Source: CAD feature listing. Evaluate the final solid. Frame: model axes, mm. A direction names the side the tool comes from. Round coordinates to 2 decimals unless told otherwise and drop trailing zeros. Order: outer loops, then holes, each group sorted by start corner. A loop starts at its lowest first (then second) coordinate and runs counter-clockwise, first axis right, second up. Notation, with made-up numbers: (79, 79.25) -> (101, 79.25) arc R26 ccw to (101, 109.25) -> close; hole circle Ø7 at (1.25, 48.5). An arc over 180 degrees is marked (long way). Use a Markdown table: item, result. Add a question column.
Autodesk Inventor part; units mm, degrees
ref_plane "YZ Plane" through (0, 0, 0) normal (1, 0, 0) x (0, 1, 0)
ref_plane "XZ Plane" through (0, 0, 0) normal (0, 1, 0) x (-1, 0, 0)
ref_plane "XY Plane" through (0, 0, 0) normal (0, 0, 1) x (1, 0, 0)
sketch "Sketch_1" plane through (0, 0, 0) normal (0, 0, 1) x (1, 0, 0)
  arc A0 (-12.6998, -10.5664) -> (-10.5664, -12.6998) centre (-10.5918, -10.5918) ccw
  arc A1 (-9.5504, -12.7) -> (-10.5664, -12.6998) centre (-10.0584, -12.7) ccw
  line L0 (-9.5504, -12.7) -> (-6.3331, -12.7)
  arc A2 (-5.3171, -12.7) -> (-6.3331, -12.7) centre (-5.8251, -12.7) ccw
  line L1 (-5.3171, -12.7) -> (-4.3434, -12.7)
  arc A3 (-4.3434, -12.7) -> (-4.3434, -10.4902) centre (-4.3434, -11.5951) ccw
  line L2 (-4.3434, -10.4902) -> (-6.4748, -10.4902)
  arc A4 (-7.1932, -8.7558) -> (-6.4748, -10.4902) centre (-6.4748, -9.4742) ccw
  line L3 (-7.1932, -8.7558) -> (-3.8632, -5.4257)
  arc A5 (-1.6181, -4.4958) -> (-3.8632, -5.4257) centre (-1.6181, -7.6708) ccw
  line L4 (-1.6181, -4.4958) -> (1.6181, -4.4958)
  arc A6 (3.8632, -5.4257) -> (1.6181, -4.4958) centre (1.6181, -7.6708) ccw
  line L5 (3.8632, -5.4257) -> (7.1932, -8.7558)
  arc A7 (6.4748, -10.4902) -> (7.1932, -8.7558) centre (6.4748, -9.4742) ccw
  line L6 (6.4748, -10.4902) -> (4.3434, -10.4902)
  arc A8 (4.3434, -10.4902) -> (4.3434, -12.7) centre (4.3434, -11.5951) ccw
  line L7 (4.3434, -12.7) -> (5.3171, -12.7)
  arc A9 (6.3331, -12.7) -> (5.3171, -12.7) centre (5.8251, -12.7) ccw
  line L8 (6.3331, -12.7) -> (9.5504, -12.7)
  arc A10 (10.5664, -12.6998) -> (9.5504, -12.7) centre (10.0584, -12.7) ccw
  arc A11 (10.5664, -12.6998) -> (12.6998, -10.5664) centre (10.5918, -10.5918) ccw
  arc A12 (12.7, -9.5504) -> (12.6998, -10.5664) centre (12.7, -10.0584) ccw
  line L9 (12.7, -9.5504) -> (12.7, -6.3331)
  arc A13 (12.7, -5.3171) -> (12.7, -6.3331) centre (12.7, -5.8251) ccw
  line L10 (12.7, -5.3171) -> (12.7, -4.3434)
  arc A14 (12.7, -4.3434) -> (10.4902, -4.3434) centre (11.5951, -4.3434) ccw
  line L11 (10.4902, -4.3434) -> (10.4902, -6.4748)
  arc A15 (8.7558, -7.1932) -> (10.4902, -6.4748) centre (9.4742, -6.4748) ccw
  line L12 (8.7558, -7.1932) -> (5.4257, -3.8632)
  arc A16 (4.4958, -1.6181) -> (5.4257, -3.8632) centre (7.6708, -1.6181) ccw
  line L13 (4.4958, -1.6181) -> (4.4958, 1.6181)
  arc A17 (5.4257, 3.8632) -> (4.4958, 1.6181) centre (7.6708, 1.6181) ccw
  line L14 (5.4257, 3.8632) -> (8.7558, 7.1932)
  arc A18 (10.4902, 6.4748) -> (8.7558, 7.1932) centre (9.4742, 6.4748) ccw
  line L15 (10.4902, 6.4748) -> (10.4902, 4.3434)
  arc A19 (10.4902, 4.3434) -> (12.7, 4.3434) centre (11.5951, 4.3434) ccw
  line L16 (12.7, 4.3434) -> (12.7, 5.3171)
  arc A20 (12.7, 6.3331) -> (12.7, 5.3171) centre (12.7, 5.8251) ccw
  line L17 (12.7, 6.3331) -> (12.7, 9.5504)
  arc A21 (12.6998, 10.5664) -> (12.7, 9.5504) centre (12.7, 10.0584) ccw
  arc A22 (12.6998, 10.5664) -> (10.5664, 12.6998) centre (10.5918, 10.5918) ccw
  arc A23 (9.5504, 12.7) -> (10.5664, 12.6998) centre (10.0584, 12.7) ccw
  line L18 (9.5504, 12.7) -> (6.3331, 12.7)
  arc A24 (5.3171, 12.7) -> (6.3331, 12.7) centre (5.8251, 12.7) ccw
  line L19 (5.3171, 12.7) -> (4.3434, 12.7)
  arc A25 (4.3434, 12.7) -> (4.3434, 10.4902) centre (4.3434, 11.5951) ccw
  line L20 (4.3434, 10.4902) -> (6.4748, 10.4902)
  arc A26 (7.1932, 8.7558) -> (6.4748, 10.4902) centre (6.4748, 9.4742) ccw
  line L21 (7.1932, 8.7558) -> (3.8632, 5.4257)
  arc A27 (1.6181, 4.4958) -> (3.8632, 5.4257) centre (1.6181, 7.6708) ccw
  line L22 (1.6181, 4.4958) -> (-1.6181, 4.4958)
  arc A28 (-3.8632, 5.4257) -> (-1.6181, 4.4958) centre (-1.6181, 7.6708) ccw
  line L23 (-3.8632, 5.4257) -> (-7.1932, 8.7558)
  arc A29 (-6.4748, 10.4902) -> (-7.1932, 8.7558) centre (-6.4748, 9.4742) ccw
  line L24 (-6.4748, 10.4902) -> (-4.3434, 10.4902)
  arc A30 (-4.3434, 10.4902) -> (-4.3434, 12.7) centre (-4.3434, 11.5951) ccw
  line L25 (-4.3434, 12.7) -> (-5.3171, 12.7)
  arc A31 (-6.3331, 12.7) -> (-5.3171, 12.7) centre (-5.8251, 12.7) ccw
  line L26 (-6.3331, 12.7) -> (-9.5504, 12.7)
  arc A32 (-10.5664, 12.6998) -> (-9.5504, 12.7) centre (-10.0584, 12.7) ccw
  arc A33 (-10.5664, 12.6998) -> (-12.6998, 10.5664) centre (-10.5918, 10.5918) ccw
  arc A34 (-12.7, 9.5504) -> (-12.6998, 10.5664) centre (-12.7, 10.0584) ccw
  line L27 (-12.7, 9.5504) -> (-12.7, 6.3331)
  arc A35 (-12.7, 5.3171) -> (-12.7, 6.3331) centre (-12.7, 5.8251) ccw
  line L28 (-12.7, 5.3171) -> (-12.7, 4.3434)
  arc A36 (-12.7, 4.3434) -> (-10.4902, 4.3434) centre (-11.5951, 4.3434) ccw
  line L29 (-10.4902, 4.3434) -> (-10.4902, 6.4748)
  arc A37 (-8.7558, 7.1932) -> (-10.4902, 6.4748) centre (-9.4742, 6.4748) ccw
  line L30 (-8.7558, 7.1932) -> (-5.4257, 3.8632)
  arc A38 (-4.4958, 1.6181) -> (-5.4257, 3.8632) centre (-7.6708, 1.6181) ccw
  line L31 (-4.4958, 1.6181) -> (-4.4958, -1.6181)
  arc A39 (-5.4257, -3.8632) -> (-4.4958, -1.6181) centre (-7.6708, -1.6181) ccw
  line L32 (-5.4257, -3.8632) -> (-8.7558, -7.1932)
  arc A40 (-10.4902, -6.4748) -> (-8.7558, -7.1932) centre (-9.4742, -6.4748) ccw
  line L33 (-10.4902, -6.4748) -> (-10.4902, -4.3434)
  arc A41 (-10.4902, -4.3434) -> (-12.7, -4.3434) centre (-11.5951, -4.3434) ccw
  line L34 (-12.7, -4.3434) -> (-12.7, -5.3171)
  arc A42 (-12.7, -6.3331) -> (-12.7, -5.3171) centre (-12.7, -5.8251) ccw
  line L35 (-12.7, -6.3331) -> (-12.7, -9.5504)
  arc A43 (-12.6998, -10.5664) -> (-12.7, -9.5504) centre (-12.7, -10.0584) ccw
  circle A44 centre (0, 0) radius 2.6035
extrude "Extrusion1" add sketch "Sketch_1" against normal blind 101.6
properties part number "1010-15-CL"
1) Section A-A on y = 0. Output: boundary loops of the cut face in (x, z).
2) Reachability of faces 1 (the cylindrical face through (2.849, -4.744, -50.089)), 2 (the flat face through (12.7, -8, -50)) from +Z, -Z, +X, -X, +Y, -Y: full face, straight path, thin tool, end or side. Return the list, or none.
3) Draft query along X for faces 3 (the cylindrical face through (7.42, 9.85, -50.09)), 4 (the flat face through (12.7, 8, -50)), 5 (the flat face through (-12.7, 8, -50)). Return one class per face: pulls with the +X half, pulls with the -X half, needs draft (parallel to the pull), parting line crosses it, or undercut.
4) Line query: probe 1 along Y at (x, z) = (7, -72); probe 2 along Y at (x, z) = (0, -26); probe 3 along X at (y, z) = (-5.25, -9). Output: solid intervals per line, ascending. Write a range as from..to.
5) First-contact query: pin 1 Ø3.5 at (y, z) = (0.5, -75) entering from +X; pin 2 Ø2.5 at (x, z) = (-0.5, -45) entering from -Y; pin 3 Ø3.5 at (y, z) = (-0.5, -40.5) entering from -X. Flat tips, straight axial feed; report the tip coordinate or a pass-through.
Conclusion:
| question | item | result |
|---|---|---|
| 1 | outline | (-4.5, -101.6) -> (-2.6, -101.6) -> (-2.6, 0) -> (-4.5, 0) -> close; (2.6, -101.6) -> (4.5, -101.6) -> (4.5, 0) -> (2.6, 0) -> close |
| 2 | face 1 | +Z, -Z |
| 2 | face 2 | +Z, -Z, +X, +Y, -Y |
| 3 | face 3 | undercut |
| 3 | face 4 | pulls with the +X half |
| 3 | face 5 | pulls with the -X half |
| 4 | probe 1 | y = -12.7..-10.34, -8.56..-5.44, 5.44..8.56, 10.34..12.7 |
| 4 | probe 2 | y = -4.5..-2.6, 2.6..4.5 |
| 4 | probe 3 | x = -12.7..-10.49, -6.81..-3.67, 3.67..6.81, 10.49..12.7 |
| 5 | pin 1 | stops at x = 4.56 |
| 5 | pin 2 | stops at y = -4.5 |
| 5 | pin 3 | stops at x = -4.56 |
